Check sheet for the modelled part. Datum: model origin and axes. Units: mm. Round coordinates to 2 decimals unless told otherwise and drop trailing zeros. Order: outer loops, then holes, each group sorted by start corner. A loop starts at its lowest first (then second) coordinate and runs counter-clockwise, first axis right, second up. Notation, with made-up numbers: (-33, 81) -> (13, 81) arc R32 cw to (13, 108) -> close; hole circle Ø2 at (-8.5, 47.25). An arc over 180 degrees is marked (long way). Answer in a Markdown table with one row per item.
```python
from build123d import *

# Parameters (mm, degrees)
SKETCH1_R           = 75
BOSS_EXTRUDE1_DEPTH = 5
CUT_EXTRUDE1_REACH  = 108.184
SKETCH2_R           = 2
CIRPATTERN1_COUNT   = 4


with BuildPart() as part:
    # Sketch1 → Boss-Extrude1 (new body)
    with BuildSketch(Plane(origin=(0, 0, 0), x_dir=(1, 0, 0), z_dir=(0, 1, 0))):
        with Locations(Location((0, 0, 0), (0, 0, 270))):
            Circle(SKETCH1_R)
    extrude(amount=BOSS_EXTRUDE1_DEPTH)

    # Sketch2 → Cut-Extrude1 (cut, up to next)
    with BuildSketch(Plane(origin=(0, 5, 0), x_dir=(1, 0, 0), z_dir=(0, 1, 0)), mode=Mode.PRIVATE) as cut_extrude1_sk1:
        with Locations(Location((0, 15, 0), (0, 0, 270))):
            Circle(SKETCH2_R)
    cut_extrude1_tool1 = extrude(cut_extrude1_sk1.sketch, amount=-CUT_EXTRUDE1_REACH, mode=Mode.PRIVATE) & part.part
    cut_extrude1 = cut_extrude1_tool1.solids().sort_by_distance((0, 5, -15))[0]
    add(cut_extrude1, mode=Mode.SUBTRACT)

    # CirPattern1: Cut-Extrude1 ×4 about axis
    cirpattern1_axis = Axis((0, 0, 0), (0, 1, 0))
    for i in range(1, CIRPATTERN1_COUNT):
        add(cut_extrude1.rotate(cirpattern1_axis, i * 360 / CIRPATTERN1_COUNT), mode=Mode.SUBTRACT)


solid = part.part
```
(1) Section check A-A on z = 0. Record the boundary of the cut face in (x, y), plus the area to 3 significant figures.
Solutions:
| item | result |
|---|---|
| outline | (-75, 0) -> (-17, 0) -> (-17, 5) -> (-75, 5) -> close; (-13, 0) -> (13, 0) -> (13, 5) -> (-13, 5) -> close; (17, 0) -> (75, 0) -> (75, 5) -> (17, 5) -> close |
| area | 710 mm^2 |
(2) Depth check by flat-ended pin: pin 1 Ø3 at (x, z) = (-15, 0) entering from +Y; pin 2 Ø3 at (y, z) = (4, -6) entering from +X; pin 3 Ø1 at (y, z) = (0.5, 50.5) entering from +X; pin 4 Ø2 at (y, z) = (3, 14) entering from +X. Enter the tip coordinate at first touch or a pass-through.
Solutions:
| item | result |
|---|---|
| pin 1 | through |
| pin 2 | x = 74.86 |
| pin 3 | x = 55.9 |
| pin 4 | x = 73.86 |
(3) Section check B-B on x = -15. Record the boundary of the cut face in (y, z).
Solutions:
| item | result |
|---|---|
| outline | (0, -73.48) -> (5, -73.48) -> (5, -2) -> (0, -2) -> close; (0, 2) -> (5, 2) -> (5, 73.48) -> (0, 73.48) -> close |
(4) Scan lines: probe 1 along Z at (x, y) = (1.5, 2.3) (3 decimals); probe 2 along Z at (x, y) = (-15, 1.8). Record each from-to range of solid material in increasing order. Write a range as from..to.
Solutions:
| item | result |
|---|---|
| probe 1 | -74.985..-16.323, -13.677..13.677, 16.323..74.985 |
| probe 2 | -73.48..-2, 2..73.48 |
(5) Section check C-C on y = 1.2. Record the boundary of the cut face in (x, z).
Solutions:
| item | result |
|---|---|
| outline | circle Ø150 at (0, 0); hole circle Ø4 at (-15, 0); hole circle Ø4 at (0, -15); hole circle Ø4 at (0, 15); hole circle Ø4 at (15, 0) |
(6) Section check D-D on z = 15. Record the boundary of the cut face in (x, y).
Solutions:
| item | result |
|---|---|
| outline | (-73.48, 0) -> (-2, 0) -> (-2, 5) -> (-73.48, 5) -> close; (2, 0) -> (73.48, 0) -> (73.48, 5) -> (2, 5) -> close |
(7) Draft check along Z on faces 1 (the flat face through (1, 5, -1)), 2 (the cylindrical face through (-1.686, 2.535, 13.925)), 3 (the cylindrical face through (-13.925, 2.535, -1.686)), 4 (the cylindrical face through (-45.636, 2.465, -59.517)). Enter one of: pulls with the +Z half, pulls with the -Z half, needs draft (parallel to the pull), parting line crosses it, or undercut.
Solutions:
| item | result |
|---|---|
| face 1 | needs draft |
| face 2 | undercut |
| face 3 | undercut |
| face 4 | parting line crosses it |
